Could you check a few things on this model? Use its own coordinates, in mm. A direction names the side the tool comes from. Round coordinates to 2 decimals unless told otherwise and drop trailing zeros. Write each loop counter-clockwise with the first axis right and the second up, starting at its lowest first coordinate (ties: lowest second). Pieces come first, ordered by that corner, then holes. Notation, with made-up numbers: (22, 71) - (67, 71) arc R19 ccw to (67, 85) - close; hole circle Ø9 at (-27.5, -31.75). An arc over 180 degrees is marked (long way). Put each result on its own line as item: value.
from build123d import *

# Parameters (mm, degrees)
F0_W     = 76.2
F0_H     = 50.8
F1_DEPTH = 5.08
F2_R     = 12.7
F3_DEPTH = 25.4
F5_DEPTH = 12.7
F6_R     = 2.38125
F7_DEPTH = 17.78
F8_R     = 2.53999


# Not quite as in the source:
# - a fillet or chamfer is up to 0.001 mm smaller than in the source, because OpenCascade refuses the exact size


with BuildPart() as f1:
    # F0 (on Front) → F1 (new body)
    with BuildSketch(Plane.XZ):
        Rectangle(F0_W, F0_H)
    extrude(amount=F1_DEPTH)

    # F2 (on face) → F3 (join)
    with BuildSketch(Plane.XZ.offset(5.08)):
        with Locations((-15.875, 2.54)):
            Circle(F2_R)
    extrude(amount=F3_DEPTH)

    # F4 (on face) → F5 (cut)
    with BuildSketch(Plane.XZ.offset(30.48)):
        Polygon((-10.31875, 5.7479024332), (-15.875, 8.9558048664), (-21.43125, 5.7479024332), (-21.43125, -0.6679024332), (-15.875, -3.8758048664), (-10.31875, -0.6679024332), align=None)
    extrude(amount=-F5_DEPTH, mode=Mode.SUBTRACT)

    # F6 (on face) → F7 (cut, through all)
    with BuildSketch(Plane.XZ.offset(17.78)):
        with Locations((-15.875, 2.54)):
            Circle(F6_R)
    extrude(amount=-F7_DEPTH, mode=Mode.SUBTRACT)

    # F8 (radius 2.54 in the source; OpenCascade refuses exactly that, so slightly less here)
    f8_edges = [f1.edges().sort_by_distance(p)[0] for p in [
        (-28.575, -30.48, 2.54),
        (-28.575, -5.08, 2.54),
        (0, -5.08, 25.4),
        (38.1, -5.08, 0),
        (0, -5.08, -25.4),
        (-38.1, -5.08, 0),
        (0, 0, -25.4),
        (-38.1, 0, 0),
        (38.1, 0, 0),
        (0, 0, 25.4),
    ]]
    fillet(f8_edges, radius=F8_R)


solid = f1.part
(1) I'm going to push flat-ended pins straight in: pin 1 (5.5 mm diameter, centred on x = -17, z = 5, fed in from -Y); pin 2 (4 mm diameter, centred on x = -21, y = -21, fed in from -Z); pin 3 (5 mm diameter, centred on x = -17, y = -9, fed in from +Z); pin 4 (4 mm diameter, centred on x = -15.875, z = 2.54, fed in from -Y). Where does each tip first touch, or does it pass through?
Values found:
pin 1: stops at y = -17.78
pin 2: stops at z = -9.77
pin 3: stops at z = 15.47
pin 4: passes through
(2) Please list where these lines run through material, in increasing order: probe 1 along Y at (x, z) = (34, 1); probe 2 along X at (y, z) = (-6.5, 3); probe 3 along X at (y, z) = (-26, 8). Write a range as from..to.
Values found:
probe 1: y = -5.08..0
probe 2: x = -28.83..-18.21, -13.54..-2.92
probe 3: x = -27.34..-17.53, -14.22..-4.41
(3) For faces 1 (the face through (0.533, -0.764, -24.676)), 2 (the face through (-21.431, -24, 3)), which set-ups out of +Z, -Z, +X, -X, +Y, -Y let a thin tool reach every point of the face, with its end or its side?
Values found:
face 1: -Z, +X, -X, +Y
face 2: -Y
(4) If we mould it in two halves opening along X, with no side actions, what happens to faces 3 (the face through (-37.376, -0.764, 0.356)), 4 (the face through (-18.614, -24.219, 7.374)), 5 (the face through (7, -5.08, 0))? For each: pulls with the +X half, pulls with the -X half, needs draft (parallel to the pull), parting line crosses it, or undercut.
Values found:
face 3: pulls with the -X half
face 4: undercut
face 5: needs draft
(5) Imagine slicing it at C-C, the plane y = -12.5. List the corners of the cut face in (x, z) for me (1 decimal), then the cut area to 3 significant figures.
Values found:
outline: circle Ø25.4 at (-15.9, 2.5); hole circle Ø4.8 at (-15.9, 2.5)
area: 489 mm^2
